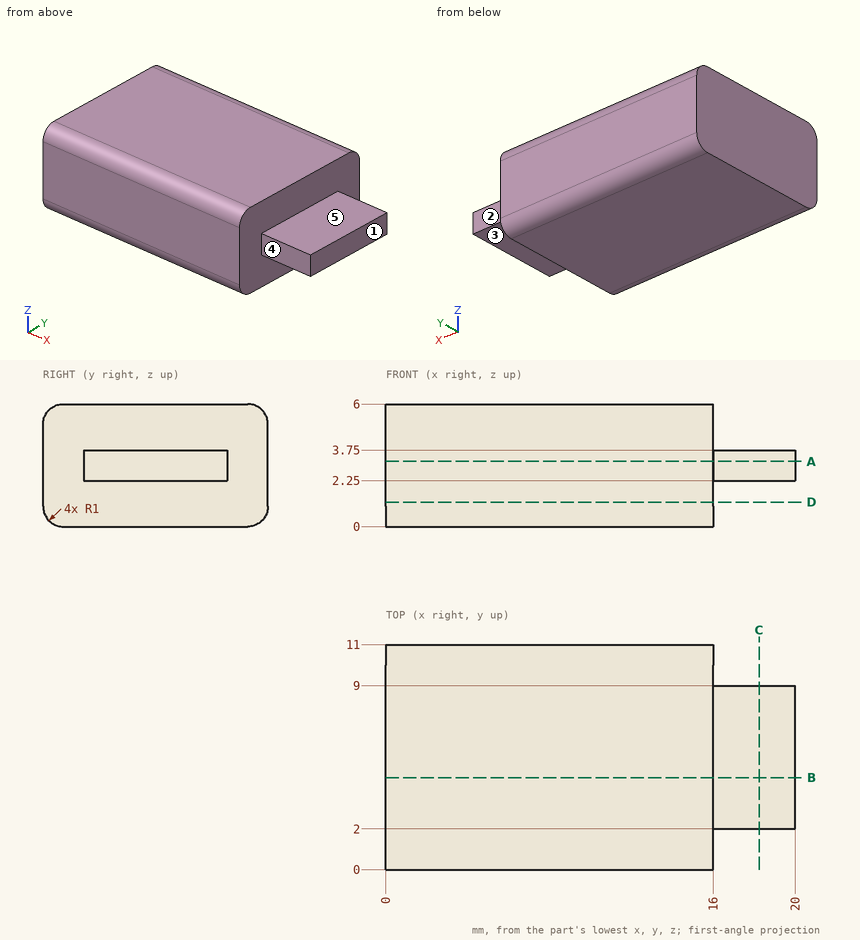
Drawing for the job (mm, zero at the part's lowest x, y, z). A direction names the side the tool comes from. Round coordinates to 2 decimals unless told otherwise and drop trailing zeros. Loops run counter-clockwise (first coordinate to the right, second up) from the corner with the lowest first, then second, coordinate; pieces in that order, holes last.
1. Band-saw the part on B-B, the plane y = 4.5. List the corners of the cut face in (x, z).
Check values:
outline: (0, 0) - (16, 0) - (16, 2.25) - (20, 2.25) - (20, 3.75) - (16, 3.75) - (16, 6) - (0, 6) - close
2. Band-saw the part on D-D, the plane z = 1.2. List the corners of the cut face in (x, y).
Check values:
outline: (0, 0) - (16, 0) - (16, 11) - (0, 11) - close
3. Band-saw the part on A-A, the plane z = 3.2. List the corners of the cut face in (x, y), and give its area (3 significant figures).
Check values:
outline: (0, 0) - (16, 0) - (16, 2) - (20, 2) - (20, 9) - (16, 9) - (16, 11) - (0, 11) - close
area: 204 mm2
4. Drop flat-ended pins along their axis: P1, Ø1.6, axis at x = 18, z = 3, coming from the +Y side; P2, Ø0.8, axis at x = 18.5, z = 3, coming from the -Y side; P3, Ø2, axis at x = 17.5, y = 5, coming from the -Z side. Give the stop position or say it passes through.
Check values:
P1: stops at y = 9
P2: stops at y = 2
P3: stops at z = 2.25
5. Band-saw the part on C-C, the plane x = 18.25. List the corners of the cut face in (y, z).
Check values:
outline: (2, 2.25) - (9, 2.25) - (9, 3.75) - (2, 3.75) - close
6. Wall check: probe 1 along Z at (x, y) = (18.75, 4.25); probe 2 along X at (y, z) = (4, 0.3); probe 3 along Y at (x, z) = (18.5, 3.6). Give the ranges that are in metal, low to high.
Check values:
probe 1: z = 2.25 to 3.75
probe 2: x = 0 to 16
probe 3: y = 2 to 9
7. Tool access for the marked faces 1, 2, 3, 4 and 5: list every direction of +Z, -Z, +X, -X, +Y, -Y with a clear straight run to the whole face (end or side of a thin tool).
Check values:
face 1: +Z, -Z, +X, +Y, -Y
face 2: +Z, -Z, +X, +Y
face 3: -Z, +X, +Y, -Y
face 4: +Z, -Z, +X, -Y
face 5: +Z, +X, +Y, -Y
